Could you check a few things on this model? Use its own coordinates, in mm. Face numbers are marked on the shaded views. A direction names the side the tool comes from. Give positions to 0.01 mm unless a question says otherwise; leave off trailing zeros. Order: outer loops, then holes, each group sorted by start corner. A loop starts at its lowest first (then second) coordinate and runs counter-clockwise, first axis right, second up. Notation, with made-up numbers: (65, -10) - (108, -10) arc R8 cw to (108, -4) - close; hole circle Ø3 at (-40, -22.75). An arc over 180 degrees is marked (long way). One line per question, with ' | ' between items. Start each with the question number.
1. I need wall thicknesses on probe 1 along Y at (x, z) = (3.3, -3.75); probe 2 along Y at (x, z) = (2.4, -4.75); probe 3 along Z at (x, y) = (-0.7, 10). Which ranges of each line are inside material? Lowest first, please. Write a range as from..to.
2. Imagine slicing it at A-A (x = 3.65). Please give me the cut outline in (y, z).
3. Imagine slicing it at B-B (y = 0.25). Please give me the cut outline in (x, z), and give its area (3 significant figures).
4. If we mould it in two halves opening along Y, with no side actions, what happens to the marked faces 1, 2, 3 and 4? For each: released by +Y, released by -Y, zero draft, split by the parting line, or undercut.
5. Imagine slicing it at C-C (x = 0.3). Please give me the cut outline in (y, z).
6. For P1, Ø2.5, axis at x = 1.5, y = 12, coming from the +Z side; P2, Ø1.6, axis at x = 2, y = 3, coming from the +Z side; P3, Ø0.9, axis at y = 2, z = -1.5, coming from the +X side; P4, Ø1.4, axis at x = 1.5, y = 0, coming from the +Z side, each with a flat end and sliding along its axis, tell me the tip position at first contact or that it passes through.
7. Which directions (+Z, -Z, +X, -X, +Y, -Y) give clear straight access to the entire face, cutting with the end or side of a thin tool? Please do the marked faces 5, 6, 7, 8 and 9.
8. Imagine slicing it at D-D (z = -4.5). Please give me the cut outline in (x, y), and give its area (3 significant figures).
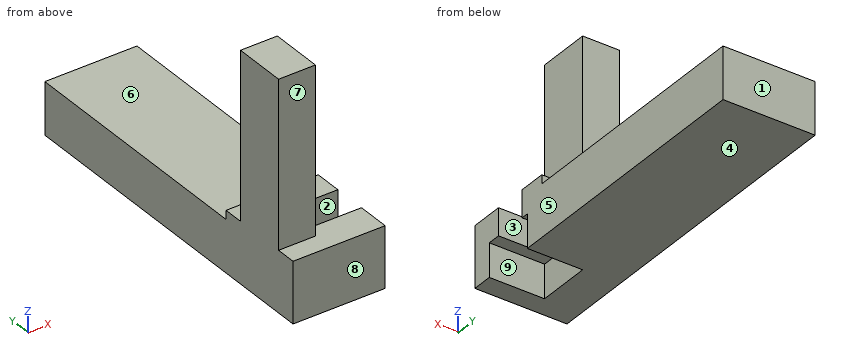
```python
from build123d import *

# Parameters (mm, degrees)
SKETCH_1_W      = 2
SKETCH_1_H      = 12
EXTRUDE_1_DEPTH = 2.9
EXTRUDE_START   = -2
SKETCH_2_W      = 1.48
SKETCH_2_H      = 1.5
SKETCH_2_H_2    = 1.8
EXTRUDE_2_DEPTH = 5
SKETCH_3_W      = 9
SKETCH_3_H      = 2.9
EXTRUDE_3_DEPTH = 2
EXTRUDE_START_2 = -5.1
SKETCH_4_W      = 2
SKETCH_4_H      = 2
EXTRUDE_4_DEPTH = 18.9
SKETCH_5_W      = 2.82
SKETCH_5_H      = 14.9
SKETCH_5_H_2    = 1.1
EXTRUDE_5_DEPTH = 5


with BuildPart() as part:
    # 草图1 → 凸台-拉伸1 (new body)
    with BuildSketch(Plane(origin=(0, 0, 0), x_dir=(1, 0, 0), z_dir=(0, 1, 0))):
        Rectangle(SKETCH_1_W, SKETCH_1_H)
    extrude(amount=EXTRUDE_1_DEPTH)

    # 草图2 → 凸台-拉伸2 (add)
    with BuildSketch(Plane(origin=(1, 0, 0), x_dir=(0, 0, -1), z_dir=(1, 0, 0)).offset(EXTRUDE_START)):
        with Locations((3.44, 3.25)):
            Rectangle(SKETCH_2_W, SKETCH_2_H)
        with Locations((3.44, -0.2)):
            Rectangle(SKETCH_2_W, SKETCH_2_H_2)
    extrude(amount=EXTRUDE_2_DEPTH)

    # 草图3 → 凸台-拉伸3 (add)
    with BuildSketch(Plane.ZY.offset(1)):
        with Locations((1.8, 1.45)):
            Rectangle(SKETCH_3_W, SKETCH_3_H)
    extrude(amount=-EXTRUDE_3_DEPTH)

    # 草图4 → 凸台-拉伸4 (add)
    with BuildSketch(Plane(origin=(0, 4, 0), x_dir=(1, 0, 0), z_dir=(0, 1, 0)).offset(EXTRUDE_START_2)):
        with Locations((0, 4.18)):
            Rectangle(SKETCH_4_W, SKETCH_4_H)
    extrude(amount=EXTRUDE_4_DEPTH)

    # 草图5 → 凸台-拉伸5 (add)
    with BuildSketch(Plane(origin=(1, 0, 0), x_dir=(0, 0, -1), z_dir=(1, 0, 0)).offset(EXTRUDE_START)):
        with Locations((4.59, 10.35)):
            Rectangle(SKETCH_5_W, SKETCH_5_H)
        with Locations((4.59, -0.55)):
            Rectangle(SKETCH_5_W, SKETCH_5_H_2)
    extrude(amount=EXTRUDE_5_DEPTH)


solid = part.part
```
Results found:
1) probe 1: y = -1.1..0.7, 2.5..17.8 | probe 2: y = -1.1..0, 2.9..17.8 | probe 3: z = -6..-3.18
2) outline: (-1.1, -6) - (0, -6) - (0, -4.18) - (0.7, -4.18) - (0.7, -2.7) - (-1.1, -2.7) - close; (2.5, -4.18) - (2.9, -4.18) - (2.9, -6) - (17.8, -6) - (17.8, -3.18) - (4, -3.18) - (4, -2.7) - (2.5, -2.7) - close
3) outline: (-1, -6) - (1, -6) - (1, -4.18) - (4, -4.18) - (4, -2.7) - (1, -2.7) - (1, 6.3) - (-1, 6.3) - close | area: 29.0 mm2
4) face 1: released by +Y | face 2: undercut | face 3: undercut | face 4: zero draft
5) outline: (-1.1, -6) - (17.8, -6) - (17.8, -3.18) - (4, -3.18) - (4, -2.7) - (2.9, -2.7) - (2.9, 6.3) - (0, 6.3) - (0, -2.7) - (-1.1, -2.7) - close
6) P1: stops at z = -3.18 | P2: stops at z = -2.7 | P3: stops at x = 1 | P4: stops at z = 6.3
7) face 5: +Z, -Z, +X, +Y, -Y | face 6: +Z, +X, -X, +Y | face 7: +Z, +X, -X, -Y | face 8: +Z, -Z, +X, -X, -Y | face 9: -Z, +X
8) outline: (-1, -1.1) - (4, -1.1) - (4, 0) - (1, 0) - (1, 2.9) - (4, 2.9) - (4, 17.8) - (-1, 17.8) - close | area: 85.8 mm2
